The model under review builds one solid part; all positions refer to its coordinate system, in mm. A direction names the side the tool comes from. Coordinates: 2 decimals unless noted, no trailing zeros. Write each loop counter-clockwise with the first axis right and the second up, starting at its lowest first coordinate (ties: lowest second). Pieces come first, ordered by that corner, then holes. Notation, with made-up numbers: (78, -37) - (97, -37) arc R23 ccw to (97, -10) - close; hole circle Ø11 at (-35.5, 32). An arc over 180 degrees is marked (long way). Put each result on its own line as item: value. Start each with the question number.
Item 1: Consider section B-B on y = 21.5. Give the boundary of the cut face in (x, z).
Item 2: Mouldability with a two-part tool opening along X and no side actions: class faces 1 (the face through (-1, 53.7, 17)), 2 (the face through (-15.786, 4.819, 0.013)), 3 (the face through (-4.01, 12.08, -18.06)) as pulls with the +X half, pulls with the -X half, needs draft (parallel to the pull), parting line crosses it, or undercut.
Item 3: Consider section C-C on z = -5. Give the boundary of the cut face in (x, y), then the cut area to 3 significant figures.
Item 4: Machinability: for faces 4 (the face through (0, -15, 9.5)), 5 (the face through (0, -21, 7)), 6 (the face through (-17, 24.5, -5)), 7 (the face through (8.97, 2.03, -12.31)), which of the approach directions +Z, -Z, +X, -X, +Y, -Y give a long, thin tool a straight path to every point of the face, cutting with its end or side? Answer none if there is none.
Item 5: For pin 1 (2 mm diameter, centred on x = 7.75, z = -13.42, fed in from +Y); pin 2 (1 mm diameter, centred on x = 0, z = -13, fed in from -Y); pin 3 (2 mm diameter, centred on x = -7.75, z = -13.42, fed in from -Y), all flat-tipped, find the tip position at first contact; note any pin that passes through.
Item 6: Consider section A-A on z = -9. Give the boundary of the cut face in (x, y), then the cut area to 3 significant figures.
Item 7: To check wall thickness, follow L1, parallel to Z at x = -7.75, y = 2.75; L2, parallel to Y at x = 8.5, z = 6; L3, parallel to Y at x = -11, z = 14. State the ranges of each line that lie inside material, in increasing order. Write a range as [from, to].
```python
from build123d import *

# Parameters (mm, degrees)
F0_R      = 18.5
F0_R_2    = 17.25
F0_R_3    = 16.7
F0_R_4    = 4.1
F1_DEPTH  = 24.5
F2_DEPTH  = 53.7
F3_R      = 16.7
F3_R_2    = 4.1
F4_DEPTH  = 1
F5_DEPTH  = 1.2
F7_D      = 3.3
F7_DEPTH  = 4
F7_TIP    = 0.9914200214
F8_DEPTH  = 21
F9_DEPTH  = 6
F11_DEPTH = 12
F13_SIZE  = 0.49999


# Not quite as in the source:
# - a fillet or chamfer is up to 0.001 mm smaller than in the source, because OpenCascade refuses the exact size
# - a feature of the source that left no trace in its solid (it failed there, or was rolled back) is left out
# - a feature names something its author has since deleted; it is built from what else it names


with BuildPart() as f1:
    # F0 (on Front) → F1 (new body)
    with BuildSketch(Plane.XZ):
        Circle(F0_R)
        Circle(F0_R_2, mode=Mode.SUBTRACT)
        Circle(F0_R_2)
        Circle(F0_R_3, mode=Mode.SUBTRACT)
        Circle(F0_R_3)
        Circle(F0_R_4, mode=Mode.SUBTRACT)
        Circle(F0_R_4)
    extrude(amount=-F1_DEPTH)

    # F0 (on Front) → F2 (join)
    with BuildSketch(Plane.XZ):
        Circle(F0_R_2)
        Circle(F0_R_3, mode=Mode.SUBTRACT)
        Circle(F0_R_3)
        Circle(F0_R_4, mode=Mode.SUBTRACT)
        Circle(F0_R_4)
    extrude(amount=-F2_DEPTH)

    # F3 (on face) → F4 (cut)
    with BuildSketch(Plane(origin=(0, 53.7, 0), x_dir=(-1, 0, 0), z_dir=(0, 1, 0))):
        Circle(F3_R)
        Circle(F3_R_2, mode=Mode.SUBTRACT)
    extrude(amount=-F4_DEPTH, mode=Mode.SUBTRACT)

    # F5 (add): a face of the model
    f5_faces = [f1.faces().sort_by_distance(p)[0] for p in [
        (0, 53.7, 0),
    ]]
    extrude(f5_faces, amount=F5_DEPTH)

    # F7
    with Locations(Plane.XZ):
        with Locations((7.75, 13.4233937587), (15.5, 0), (7.75, -13.4233937587), (-7.75, -13.4233937587), (-15.5, 0), (-7.75, 13.4233937587)):
            Hole(F7_D / 2, depth=F7_DEPTH)
            with Locations((0, 0, -(F7_DEPTH + F7_TIP / 2))):  # 118° drill point
                Cone(0, F7_D / 2, F7_TIP, mode=Mode.SUBTRACT)

    # F6 (on face) → F8 (join)
    with BuildSketch(Plane.XZ):
        with BuildLine():
            ThreePointArc((0.5863406929, 4.0578571429), (0, 4.1), (-0.5863406929, 4.0578571429))
            ThreePointArc((-0.5863406929, 4.0578571429), (0, 4), (0.5863406929, 4.0578571429))
        make_face()
        with BuildLine():
            ThreePointArc((-1.6583123952, 9.5), (-2.9434412837, 6.4202126173), (-0.5863406929, 4.0578571429))
            ThreePointArc((-0.5863406929, 4.0578571429), (0, 4.1), (0.5863406929, 4.0578571429))
            ThreePointArc((0.5863406929, 4.0578571429), (2.3193772956, 5.0972417493), (3, 7))
            ThreePointArc((3, 7), (2.6433820369, 8.4186371655), (1.6583123952, 9.5))
            Line((1.6583123952, 9.5), (-1.6583123952, 9.5))
        make_face()
        with BuildLine():
            ThreePointArc((1.6583123952, 9.5), (0, 10), (-1.6583123952, 9.5))
            Line((-1.6583123952, 9.5), (1.6583123952, 9.5))
        make_face()
    extrude(amount=F8_DEPTH)

    # F6 (on face) → F9 (join)
    with BuildSketch(Plane.XZ):
        with BuildLine():
            ThreePointArc((-0.5863406929, 4.0578571429), (-2.2505108877, 3.4271271853), (-3.4906475169, 2.1506696429))
            ThreePointArc((-3.4906475169, 2.1506696429), (0, 1.025), (3.4906475169, 2.1506696429))
            ThreePointArc((3.4906475169, 2.1506696429), (2.2505108877, 3.4271271853), (0.5863406929, 4.0578571429))
            ThreePointArc((0.5863406929, 4.0578571429), (0, 4), (-0.5863406929, 4.0578571429))
        make_face()
        with BuildLine():
            ThreePointArc((3.4906475169, 2.1506696429), (5.3177647519, 4.2756646603), (5.975, 7))
            ThreePointArc((5.975, 7), (-2.7243353397, 12.3177647519), (-3.4906475169, 2.1506696429))
            ThreePointArc((-3.4906475169, 2.1506696429), (-2.2505108877, 3.4271271853), (-0.5863406929, 4.0578571429))
            ThreePointArc((-0.5863406929, 4.0578571429), (-2.9434412837, 6.4202126173), (-1.6583123952, 9.5))
            ThreePointArc((-1.6583123952, 9.5), (0, 10), (1.6583123952, 9.5))
            ThreePointArc((1.6583123952, 9.5), (2.6433820369, 8.4186371655), (3, 7))
            ThreePointArc((3, 7), (2.3193772956, 5.0972417493), (0.5863406929, 4.0578571429))
            ThreePointArc((0.5863406929, 4.0578571429), (2.2505108877, 3.4271271853), (3.4906475169, 2.1506696429))
        make_face()
    extrude(amount=F9_DEPTH)

    # F10 (on face) → F11 (cut)
    with BuildSketch(Plane.XZ.offset(21)):
        with BuildLine():
            ThreePointArc((1.6583123952, 9.5), (0, 10), (-1.6583123952, 9.5))
            Line((-1.6583123952, 9.5), (1.6583123952, 9.5))
        make_face()
    extrude(amount=-F11_DEPTH, mode=Mode.SUBTRACT)

    # F13 (size 0.5 in the source; OpenCascade refuses exactly that, so slightly less here)
    f13_edges = [f1.edges().sort_by_distance(p)[0] for p in [
        (-3.490648, -6, 11.84933),
        (0, -21, 4),
    ]]
    chamfer(f13_edges, length=F13_SIZE)


solid = f1.part
```
Report:
1. outline: circle Ø37 at (0, 0)
2. face 1: needs draft
2. face 2: undercut
2. face 3: parting line crosses it
3. outline: (-17.81, 0) - (17.81, 0) - (17.81, 24.5) - (16.51, 24.5) - (16.51, 53.7) - (15.93, 53.7) - (15.93, 52.7) - (-15.93, 52.7) - (-15.93, 53.7) - (-16.51, 53.7) - (-16.51, 24.5) - (-17.81, 24.5) - close
3. area: 1,810 mm²
4. face 4: +Z, +X, -X, -Y
4. face 5: +Z, -Z, +X, -X, -Y
4. face 6: +Y
4. face 7: -Y
5. pin 1: y = 52.7
5. pin 2: y = 0
5. pin 3: y = 4.39
6. outline: (-16.16, 0) - (16.16, 0) - (16.16, 24.5) - (14.72, 24.5) - (14.72, 53.7) - (14.07, 53.7) - (14.07, 52.7) - (-14.07, 52.7) - (-14.07, 53.7) - (-14.72, 53.7) - (-14.72, 24.5) - (-16.16, 24.5) - close
6. area: 1,620 mm²
7. L1: [-16.8, -15.07], [-11.77, 11.77], [15.07, 16.8]
7. L2: [0, 52.7]
7. L3: [0, 24.5]
